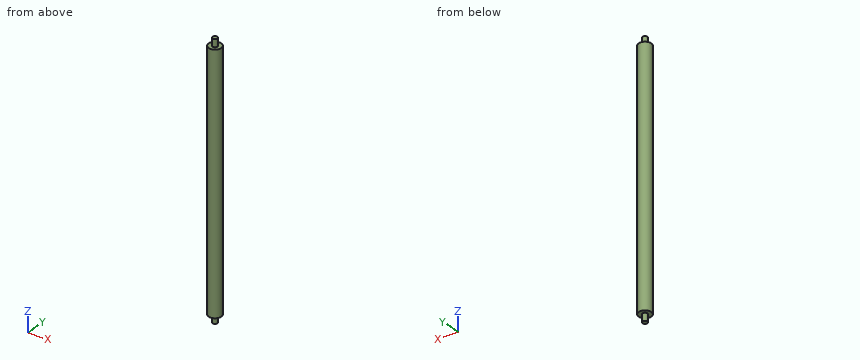
Autodesk Inventor part; units mm, degrees
ref_plane "YZ Plane" through (0, 0, 0) normal (1, 0, 0) x (0, 1, 0)
ref_plane "XZ Plane" through (0, 0, 0) normal (0, 1, 0) x (-1, 0, 0)
ref_plane "XY Plane" through (0, 0, 0) normal (0, 0, 1) x (1, 0, 0)
sketch "Sketch1" plane through (0, 0, 0) normal (0, 0, 1) x (1, 0, 0)
  circle A0 centre (0, 0) radius 2.5
  dimension "d0" = 5
extrude "Extrusion1" add sketch "Sketch1" along normal blind 100
sketch "Sketch2" plane through (0, 0, 100) normal (0, 0, 1) x (1, 0, 0)
  circle A0 centre (0, 0) radius 2.5
  circle A1 centre (0, 0) radius 1
  dimension "d3" = 2
extrude "Extrusion2" add sketch "Sketch2" along normal blind 3 contours A1
sketch "Sketch3" plane through (0, 0, 0) normal (0, 0, -1) x (-1, 0, 0)
  circle A0 centre (0, 0) radius 1
  dimension "d6" = 2
extrude "Extrusion3" add sketch "Sketch3" along normal blind 3
properties part number "Bone-10cm"
Model file for the job. Use its own axes, mm. Give positions to 0.01 mm unless a question says otherwise; leave off trailing zeros. Loops run counter-clockwise (first coordinate to the right, second up) from the corner with the lowest first, then second, coordinate; pieces in that order, holes last.
1) Saw through at C-C (z = 70). Write the cut outline in (x, y), plus the area to 3 significant figures.
2) Wall check: line 1 (X direction, y = -0.25, z = 19.5); line 2 (Z direction, x = 1, y = 2.1); line 3 (X direction, y = -2.3, z = 13). Give the ranges that are in metal, low to high.
3) Saw through at A-A (y = 0). Write the cut outline in (x, z).
4) Flat gauge pins, fed straight in: pin 1 Ø1 at (y, z) = (-1, 65) entering from +X; pin 2 Ø1 at (x, y) = (-2, -1.5) entering from +Z; pin 3 Ø2 at (x, y) = (-2, 0.5) entering from -Z. Where does each tip first touch, or does it go through?
Answer block:
1. outline: circle Ø5 at (0, 0)
1. area: 19.6 mm2
2. line 1: x = -2.49 to 2.49
2. line 2: z = 0 to 100
2. line 3: x = -0.98 to 0.98
3. outline: (-2.5, 0) - (-1, 0) - (-1, -3) - (1, -3) - (1, 0) - (2.5, 0) - (2.5, 100) - (1, 100) - (1, 103) - (-1, 103) - (-1, 100) - (-2.5, 100) - close
4. pin 1: stops at x = 2.45
4. pin 2: stops at z = 100
4. pin 3: stops at z = 0
